Geometry check sheet. Reference: the model listing, model coordinates, mm. A direction names the side the tool comes from. Give positions to 0.01 mm unless a question says otherwise; leave off trailing zeros. Write each loop counter-clockwise with the first axis right and the second up, starting at its lowest first coordinate (ties: lowest second). Pieces come first, ordered by that corner, then holes. Notation, with made-up numbers: M -8,41 L -1,41 A6 ccw -1,47 Z; hole C 52,27 d10. An arc over 180 degrees is marked long. One line per item, written item: value. Start each with the question number.
1. Cross-section at D-D on x = 71.5. Record the cut outline in (y, z).
2. Cross-section at C-C on z = 39. Count the separate pieces of the cut face and the enclosed holes in it, then the cut area to 3 significant figures.
3. Gauge pin test, flat ends, axial feed: pin 1 (13.5 mm diameter, centred on y = -10.5, z = 88, fed in from -X); pin 2 (12 mm diameter, centred on y = -14.5, z = 116, fed in from -X); pin 3 (3.5 mm diameter, centred on y = -8, z = 230, fed in from -X). Record the tip position at first contact, or that the pin passes through.
4. Tool access check on faces 5 (the face through (240.57, -13, 72)), 6 (the face through (22.31, -13, 91)), 7 (the face through (51.48, -12.52, 84.56)). Record the directions out of +Z, -Z, +X, -X, +Y, -Y that give a thin tool (end or side, any length) a straight path to the whole face; none if there is none.
5. Release check for a two-part mould opening along X. For faces 1 (the face through (141.534, -12.629, 234.382)), 2 (the face through (221.658, -12.522, 162.637)), 3 (the face through (127, 0, 121)), 4 (the face through (44.044, -12.522, 15.099)) record: pulls with the +X half, pulls with the -X half, needs draft (parallel to the pull), parting line crosses it, or undercut.
6. Scan lines: line 1 (X direction, y = -16.25, z = 52.5); line 2 (Z direction, x = 230, y = -3.25); line 3 (X direction, y = -11.25, z = 112). Record each from-to range of solid material in increasing order.
7. Cross-section at B-B on z = 133. Record the cut outline in (x, y), then the cut area to 3 significant figures.
8. Cross-section at A-A on x = 100. Record the cut outline in (y, z).
from build123d import *

# Parameters (mm, degrees)
F1_DEPTH = 25.4
F3_DEPTH = 25.4
F5_DEPTH = 7.62
F7_DEPTH = 7.62


with BuildPart() as f1:
    # F0 (on Front) → F1 (new body)
    with BuildSketch(Plane.XZ):
        with BuildLine():
            ThreePointArc((55.4591871163, 137.7187907169), (57.1778936646, 140.1694279188), (59.0786326768, 142.4817354462))
            ThreePointArc((59.0786326768, 142.4817354462), (39.0356978447, 161.9894984881), (18.9927630126, 142.4817354462))
            ThreePointArc((18.9927630126, 142.4817354462), (15.5809128086, 125.4101537656), (18.9927630126, 108.3385720849))
            Line((18.9927630126, 108.3385720849), (22.309999913, 97.1100777388))
            Line((22.309999913, 97.1100777388), (22.309999913, 84.7518071532))
            Line((22.309999913, 84.7518071532), (33.4528027138, 104.264870286))
            Line((33.4528027138, 104.264870286), (33.4528027138, 86.6916491587))
            Line((33.4528027138, 86.6916491587), (36.9130928491, 112.466349486))
            Line((36.9130928491, 112.466349486), (43.123934418, 97.1100777388))
            ThreePointArc((43.123934418, 97.1100777388), (41.9493193566, 113.4261599819), (37.8830172122, 129.2710155249))
            ThreePointArc((37.8830172122, 129.2710155249), (41.7069327363, 143.8231946906), (55.4591871163, 137.7187907169))
        make_face()
        with BuildLine():
            Line((161.0753406305, 231.77226012), (157.3511064053, 226.7855703831))
            Line((157.3511064053, 226.7855703831), (153.2667279243, 222.1906334162))
            Line((153.2667279243, 222.1906334162), (135.5471188815, 203.6892712114))
            ThreePointArc((135.5471188815, 203.6892712114), (124.4679795229, 189.3777542773), (142.5452232361, 188.4945183992))
            Line((142.5452232361, 188.4945183992), (157.3511064053, 188.4945183992))
            ThreePointArc((157.3511064053, 188.4945183992), (163.0913283676, 173.9439144731), (157.3511064053, 159.3933105469))
            ThreePointArc((157.3511064053, 159.3933105469), (133.5218764448, 146.628732852), (106.8485764131, 151.0221039559))
            ThreePointArc((106.8485764131, 151.0221039559), (81.4826477265, 155.0355463169), (59.0786326768, 142.4817354462))
            ThreePointArc((59.0786326768, 142.4817354462), (57.1778936646, 140.1694279188), (55.4591871163, 137.7187907169))
            ThreePointArc((55.4591871163, 137.7187907169), (49.1972996165, 115.7594263547), (56.2388920861, 94.0375274104))
            ThreePointArc((56.2388920861, 94.0375274104), (51.4005357949, 84.435997918), (44.5201359689, 76.1740878224))
            ThreePointArc((44.5201359689, 76.1740878224), (33.1757105593, 71.4588467738), (31.2459021807, 59.3260265887))
            ThreePointArc((31.2459021807, 59.3260265887), (28.0144474885, 44.7267728634), (21.5454995632, 31.2459263951))
            ThreePointArc((21.5454995632, 31.2459263951), (25.0258299967, 19.4454210796), (26.6509782523, 7.2501958348))
            Line((26.6509782523, 7.2501958348), (45.5412305892, 7.2501958348))
            ThreePointArc((45.5412305892, 7.2501958348), (43.9865002742, 15.1994537749), (37.8830172122, 20.52443102))
            ThreePointArc((37.8830172122, 20.52443102), (39.9724122876, 31.2459263951), (37.8830172122, 41.9674217701))
            ThreePointArc((37.8830172122, 41.9674217701), (43.3657124777, 53.2576823746), (51.4005357949, 62.8998577595))
            ThreePointArc((51.4005357949, 62.8998577595), (63.9434482796, 70.1826306752), (75.6635218859, 78.7268280983))
            ThreePointArc((75.6635218859, 78.7268280983), (79.7479003668, 78.2162845135), (83.8322788477, 78.7268280983))
            ThreePointArc((83.8322788477, 78.7268280983), (80.62219761, 70.8415194676), (75.6635218859, 63.9209523797))
            ThreePointArc((75.6635218859, 63.9209523797), (94.8811032097, 51.3116760169), (110.8912838002, 34.8197567898))
            Line((110.8912838002, 34.8197567898), (118.0389523506, 23.5877130181))
            ThreePointArc((118.0389523506, 23.5877130181), (122.7991958663, 28.8657998516), (124.165520072, 35.8408465981))
            ThreePointArc((124.165520072, 35.8408465981), (117.7349645729, 43.3549786498), (114.4651249051, 52.6889152825))
            ThreePointArc((114.4651249051, 52.6889152825), (101.2536184714, 56.1015596962), (93.0221304297, 66.9842362404))
            ThreePointArc((93.0221304297, 66.9842362404), (105.7958752022, 76.2573128263), (114.4651249051, 89.4483178854))
            ThreePointArc((114.4651249051, 89.4483178854), (137.6729881459, 85.3431639936), (161.1937859731, 86.8362394266))
            Line((161.1937859731, 86.8362394266), (161.1937859731, 60.947837063))
            add(Edge.make_bspline(
                [(161.1937859731, 60.947837063), (157.8993693687, 59.0561358776), (150.6323180509, 54.8832909577), (162.2144334117, 39.9763215602), (143.2040633117, 24.6385665246), (159.3573781955, 18.7003155427), (150.8482458466, 9.9391907933), (152.7499995265, 7.8050355296)],
                knots=[0, 0, 0, 0, 0.0779334272, 0.1719109278, 0.2757758884, 0.3531240541, 0.4319815568, 0.4319815568, 0.4319815568, 0.4319815568], degree=3))
            Line((152.7499995265, 7.8050355296), (173.171891931, 9.0224858617))
            ThreePointArc((173.171891931, 9.0224858617), (172.9779809567, 10.1232568284), (172.664853356, 11.1962196856))
            add(Edge.make_bspline(
                [(172.664853356, 11.1962196856), (171.3313436819, 12.7085104711), (168.5824067748, 14.597468285), (167.0453242097, 17.1912484114)],
                knots=[0.5736467919, 0.5736467919, 0.5736467919, 0.5736467919, 0.6257117477, 0.6257117477, 0.6257117477, 0.6257117477], degree=3))
            add(Edge.make_bspline(
                [(167.0453242097, 17.1912484114), (166.5426299969, 18.0395296218), (166.169553332, 18.9631972351), (165.9011092746, 19.9468993754)],
                knots=[0.6257117477, 0.6257117477, 0.6257117477, 0.6257117477, 0.6427392989, 0.6427392989, 0.6427392989, 0.6427392989], degree=3))
            ThreePointArc((165.9011092746, 19.9468993754), (164.2768081704, 31.0782012829), (167.0453242097, 41.9813914203))
            add(Edge.make_bspline(
                [(167.0453242097, 41.9813914203), (167.3962963394, 49.2992780507), (165.4846355858, 55.0477309675), (167.0453242097, 61.3542387283)],
                knots=[0.7506807864, 0.7506807864, 0.7506807864, 0.7506807864, 0.8611546748, 0.8611546748, 0.8611546748, 0.8611546748], degree=3))
            add(Edge.make_bspline(
                [(167.0453242097, 61.3542387283), (169.0068222846, 69.2803571375), (176.4531944079, 78.0879710988), (183.8995665312, 86.8955850601)],
                knots=[0.8611546748, 0.8611546748, 0.8611546748, 0.8611546748, 1, 1, 1, 1], degree=3))
            ThreePointArc((183.8995665312, 86.8955850601), (200.6813055662, 83.248064902), (217.7208593273, 85.3892738977))
            ThreePointArc((217.7208593273, 85.3892738977), (229.8786920932, 81.8087152157), (231.4277632013, 69.2296183983))
            Line((231.4277632013, 69.2296183983), (228.5562352695, 63.4104087949))
            Line((228.5562352695, 63.4104087949), (231.4277632013, 57.001966241))
            Line((231.4277632013, 57.001966241), (221.0727564471, 52.3620415043))
            Line((221.0727564471, 52.3620415043), (222.7011620998, 44.7454368664))
            Line((222.7011620998, 44.7454368664), (237.3357014598, 47.8742544631))
            Line((237.3357014598, 47.8742544631), (240.5703216791, 63.4104087949))
            Line((240.5703216791, 63.4104087949), (240.5703216791, 81.790111959))
            ThreePointArc((240.5703216791, 81.790111959), (237.5070340931, 96.5959839523), (222.7011620998, 99.6592715383))
            Line((222.7011620998, 99.6592715383), (208.9163959026, 107.8280285001))
            ThreePointArc((208.9163959026, 107.8280285001), (216.2226754166, 127.6019199845), (215.5535072088, 148.6718207598))
            ThreePointArc((215.5535072088, 148.6718207598), (218.0854842896, 143.9483475476), (222.190618515, 140.503063798))
            ThreePointArc((222.190618515, 140.503063798), (220.0514151702, 151.3432226251), (215.5535072088, 161.4354997873))
            Line((215.5535072088, 161.4354997873), (229.0830209851, 152.8838410974))
            Line((229.0830209851, 152.8838410974), (214.0218615532, 172.6675480604))
            Line((214.0218615532, 172.6675480604), (219.6378856897, 172.6675480604))
            Line((219.6378856897, 172.6675480604), (208.4058374166, 184.6981031667))
            Line((208.4058374166, 184.6981031667), (213.5113179684, 186.4523291588))
            Line((213.5113179684, 186.4523291588), (208.4058374166, 201.3112651118))
            Line((208.4058374166, 201.3112651118), (213.5113179684, 201.7687410116))
            Line((213.5113179684, 201.7687410116), (200.6355195315, 214.0218764544))
            Line((200.6355195315, 214.0218764544), (208.4058374166, 213.5113328695))
            ThreePointArc((208.4058374166, 213.5113328695), (200.6355195315, 219.8232430535), (191.0472214222, 222.7011919022))
            ThreePointArc((191.0472214222, 222.7011919022), (182.6973201136, 228.8132361759), (172.5500786904, 226.7855703831))
            Line((172.5500786904, 226.7855703831), (167.7524379956, 231.3804924488))
            Line((167.7524379956, 231.3804924488), (167.7524379956, 226.7855703831))
            Line((167.7524379956, 226.7855703831), (161.0753406305, 231.77226012))
        make_face()
    extrude(amount=F1_DEPTH)

    # F2 (on Front) → F3 (join)
    with BuildSketch(Plane.XZ):
        Polygon((130.7088136673, 246.8455582857), (152.7369320393, 221.4836478233), (157.5240641832, 226.5485674143), align=None)
    extrude(amount=F3_DEPTH)

    # F4 (on face) → F5 (cut)
    with BuildSketch(Plane(origin=(0, 0, 0), x_dir=(-1, 0, 0), z_dir=(0, 1, 0))):
        Polygon((-157.2947343563, 226.7221516738), (-152.6668710263, 221.5643120502), (-130.7088136673, 246.8455582857), align=None)
    extrude(amount=-F5_DEPTH, mode=Mode.SUBTRACT)

    # F6 (on face) → F7 (cut)
    with BuildSketch(Plane.XZ.offset(25.4)):
        Polygon((130.7088136673, 246.8455582857), (152.6668710263, 221.5643120502), (157.2944223706, 226.7223878219), align=None)
    extrude(amount=-F7_DEPTH, mode=Mode.SUBTRACT)


solid = f1.part
Report:
1. outline: M -25.4,75.48 L 0,75.48 L 0,151.83 L -25.4,151.83 Z
2. separate pieces: 3
2. enclosed holes: 0
2. area: 913 mm^2
3. pin 1: stops at x = 22.31
3. pin 2: stops at x = 15.71
3. pin 3: stops at x = 143.82
4. face 5: -Z, +X, +Y, -Y
4. face 6: -X, +Y, -Y
4. face 7: +Y, -Y
5. face 1: pulls with the -X half
5. face 2: pulls with the +X half
5. face 3: needs draft
5. face 4: undercut
6. line 1: x = 30.17 to 42.89, 93.42 to 114.49, 154.38 to 166.56, 221.38 to 238.3
6. line 2: z = 46.31 to 56.36, 60.19 to 66.34, 81.66 to 100.45
6. line 3: x = 17.65 to 36.85, 37.1 to 42.17, 49.45 to 211.21
7. outline: M 16.23,-25.4 L 36.3,-25.4 L 36.3,0 L 16.23,0 Z; M 52.85,-25.4 L 216.83,-25.4 L 216.83,0 L 52.85,0 Z
7. area: 4,670 mm^2
8. outline: M -25.4,46.79 L 0,46.79 L 0,57.01 L -25.4,57.01 Z; M -25.4,71.17 L 0,71.17 L 0,153.88 L -25.4,153.88 Z
